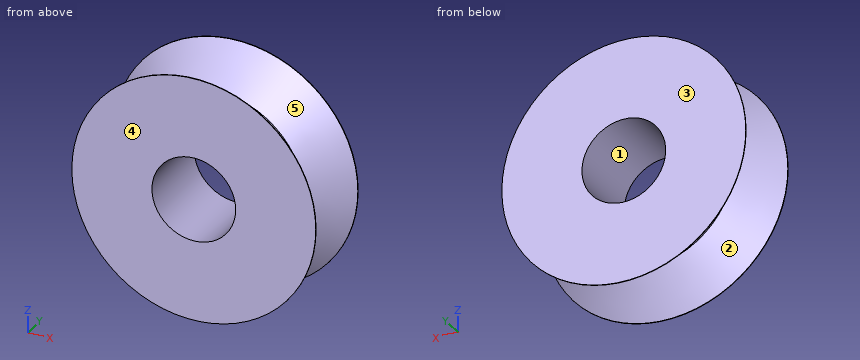
from build123d import *

# Parameters (mm, degrees)
SKETCH7_R          = 6.5405
CUT_EXTRUDE2_DEPTH = 13.7


with BuildPart() as part:
    # Sketch2 → Revolve1 (revolve)
    with BuildSketch(Plane.XY):
        Polygon((0, 0), (19.05, 0), (19.05, 0.1), (13.59375, 5.55625), (13.59375, 7.14375), (19.05, 12.6), (19.05, 12.7), (0, 12.7), align=None)
    revolve(axis=Axis((0, 0, 0), (0, 1, 0)))

    # Sketch7 → Cut-Extrude2 (cut, through all)
    with BuildSketch(Plane(origin=(0, 12.7, 0), x_dir=(1, 0, 0), z_dir=(0, 1, 0))):
        Circle(SKETCH7_R)
    extrude(amount=-CUT_EXTRUDE2_DEPTH, mode=Mode.SUBTRACT)


solid = part.part
Read the model definition and answer for the solid it produces. Units are mm, in the model's axes. Face numbers are marked on the shaded views. A direction names the side the tool comes from. Coordinates: 2 decimals unless noted, no trailing zeros. Write each loop counter-clockwise with the first axis right and the second up, starting at its lowest first coordinate (ties: lowest second). Pieces come first, ordered by that corner, then holes. Notation, with made-up numbers: M 30.5,57.25 L 44.5,57.25 A18 ccw 44.5,72.25 Z; hole C 87,-2.75 d11. An arc over 180 degrees is marked long. Use a Markdown table: item, result.
Q1. The part is cut by section C-C, the plane y = 9.5. Write down the section's boundary in (x, z), then the cut area to 3 significant figures.
Answer block:
| item | result |
|---|---|
| outline | C 0,0 d31.9; hole C 0,0 d13.08 |
| area | 665 mm2 |
Q2. The part is cut by section D-D, the plane y = 6.5. Write down the section's boundary in (x, z).
Answer block:
| item | result |
|---|---|
| outline | C 0,0 d27.19; hole C 0,0 d13.08 |
Q3. Straight lines are drawn through the part: L1, parallel to X at y = 3.25, z = 0; L2, parallel to Z at x = 0, y = 9; L3, parallel to Y at x = -14, z = -10.5. For each, find the intervals that lie inside material, in ascending order. Write a range as [from, to].
Answer block:
| item | result |
|---|---|
| L1 | x = [-15.9, -6.54], [6.54, 15.9] |
| L2 | z = [-15.45, -6.54], [6.54, 15.45] |
| L3 | y = [0, 1.65], [11.05, 12.7] |
Q4. Each of these flat-tipped pins is pushed along its axis until it touches: pin 1 Ø5 at (x, y) = (-10.5, 7.5) entering from +Z; pin 2 Ø6 at (y, z) = (3, -0.5) entering from +X; pin 3 Ø3 at (y, z) = (3.5, -5.5) entering from +X; pin 4 Ø1 at (x, y) = (10.5, 6.5) entering from -Z. Where does it stop, or does it pass through?
Answer block:
| item | result |
|---|---|
| pin 1 | stops at z = 13.2 |
| pin 2 | stops at x = 19.05 |
| pin 3 | stops at x = 16.32 |
| pin 4 | stops at z = -9.21 |
Q5. Determine the mould class of the marked faces 1, 2 and 3 for opening direction Y: released by +Y, released by -Y, zero draft, split by the parting line, or undercut.
Answer block:
| item | result |
|---|---|
| face 1 | zero draft |
| face 2 | undercut |
| face 3 | released by +Y |
Q6. The part is cut by section A-A, the plane z = 0. Write down the section's boundary in (x, y).
Answer block:
| item | result |
|---|---|
| outline | M -19.05,0 L -6.54,0 L -6.54,12.7 L -19.05,12.7 L -19.05,12.6 L -13.59,7.14 L -13.59,5.56 L -19.05,0.1 Z; M 6.54,0 L 19.05,0 L 19.05,0.1 L 13.59,5.56 L 13.59,7.14 L 19.05,12.6 L 19.05,12.7 L 6.54,12.7 Z |
Q7. Which of the six approach directions +Z, -Z, +X, -X, +Y, -Y give full straight-line access (tool end or side, diameter ignored) to the marked faces 4 and 5?
Answer block:
| item | result |
|---|---|
| face 4 | +Z, -Z, +X, -X, -Y |
| face 5 | none |
Q8. The part is cut by section B-B, the plane x = 0. Write down the section's boundary in (y, z), then the cut area to 3 significant figures.
Answer block:
| item | result |
|---|---|
| outline | M 0,-19.05 L 0.1,-19.05 L 5.56,-13.59 L 7.14,-13.59 L 12.6,-19.05 L 12.7,-19.05 L 12.7,-6.54 L 0,-6.54 Z; M 0,6.54 L 12.7,6.54 L 12.7,19.05 L 12.6,19.05 L 7.14,13.59 L 5.56,13.59 L 0.1,19.05 L 0,19.05 Z |
| area | 241 mm2 |
